from build123d import *

# Parameters (mm, degrees)
F0_R     = 4.7625
F0_R_2   = 1.27
F1_DEPTH = 3.175
F2_R     = 12.7


with BuildPart() as f1:
    # F0 (on Front) → F1 (new body, symmetric)
    with BuildSketch(Plane.XZ):
        with BuildLine():
            ThreePointArc((-58.739439, 25.245564), (-67.461813, 27.891467), (-61.679409, 20.845588))
            ThreePointArc((-61.679409, 20.845588), (-59.542065, 22.599661), (-58.739439, 25.245564))
        make_face()
        Polygon((-45.276641, -18.754199), (0, 0), (0, 80.759988), (-139.00587, 23.181871), (-110.452903, -45.75109), align=None)
        with Locations((-91.447397, -8.667692)):
            Circle(F0_R, mode=Mode.SUBTRACT)
        with Locations((-96.914986, 4.532236)):
            Circle(F0_R_2, mode=Mode.SUBTRACT)
        with BuildLine():
            ThreePointArc((-56.764349, 12.045635), (-56.978383, 11.340061), (-57.548342, 10.872308))
            ThreePointArc((-57.548342, 10.872308), (-59.207676, 11.559627), (-58.520357, 13.218962))
            ThreePointArc((-58.520357, 13.218962), (-57.328775, 13.101602), (-56.764349, 12.045635))
        make_face(mode=Mode.SUBTRACT)
        with BuildLine():
            ThreePointArc((-58.739439, 25.245564), (-59.542065, 22.599661), (-61.679409, 20.845588))
            ThreePointArc((-61.679409, 20.845588), (-67.461813, 27.891467), (-58.739439, 25.245564))
        make_face(mode=Mode.SUBTRACT)
        Polygon((0, 80.759988), (0, 0), (110.452903, -45.75109), (139.00587, 23.181871), align=None)
        with Locations((58.034349, 12.045635)):
            Circle(F0_R_2, mode=Mode.SUBTRACT)
        with Locations((91.447397, -8.667692)):
            Circle(F0_R, mode=Mode.SUBTRACT)
        with Locations((96.914986, 4.532236)):
            Circle(F0_R_2, mode=Mode.SUBTRACT)
        with Locations((63.501939, 25.245564)):
            Circle(F0_R, mode=Mode.SUBTRACT)
    extrude(amount=F1_DEPTH, both=True)

    # F2
    f2_edges = [f1.edges().sort_by_distance(p)[0] for p in [
        (-139.00587, 0, 23.181871),
        (0, 0, 80.759988),
        (0, 0, 0),
        (110.452903, 0, -45.75109),
        (139.00587, 0, 23.181871),
        (-110.452903, 0, -45.75109),
    ]]
    fillet(f2_edges, radius=F2_R)


solid = f1.part
For this review, take the finished solid that the model builds, in its own axes (mm). A direction names the side the tool comes from. Round coordinates to 2 decimals unless told otherwise and drop trailing zeros. Loops run counter-clockwise (first coordinate to the right, second up) from the corner with the lowest first, then second, coordinate; pieces in that order, holes last. Notation, with made-up numbers: (32.25, 9) - (57.25, 9) arc R24 ccw to (57.25, 46) - close; hole circle Ø11 at (43, 52). An arc over 180 degrees is marked (long way). Put each result on its own line as item: value. Start each with the question number.
1. Consider section B-B on z = 37.5. State the section outline as (x, y) points (3 decimals), plus the area to 3 significant figures.
2. Insertion check: P1, Ø1.5, axis at x = -96.91, z = 4.53, coming from the -Y side; P2, Ø12.5, axis at x = -63.5, z = 25.25, coming from the -Y side (3 decimals); P3, Ø1.5, axis at x = 59.5, y = 0.5, coming from the +Z side; P4, Ø1.5, axis at y = -0.5, z = 65.5, coming from the -X side. Each pin has a flat end and moves straight along its axis. Give the tip position at first contact, or say it passes through.
3. For faces 5 (the cylindrical face through (-134.2, 0.04, 21.04)), 6 (the flat face through (51.13, -0.04, -21.18)), list the 3-axis set-ups (+Z, -Z, +X, -X, +Y, -Y) from which the entire face can be reached by the end or side of a thin tool; tool diameter is ignored.
4. For probe 1 along X at (y, z) = (2.5, -5); probe 2 along X at (y, z) = (0.5, -22); probe 3 along Z at (x, y) = (9.5, 2), list the stretches that pass through material, from the lowest coordinate up. Write a range as [from, to].
5. Consider section C-C on x = 48. State the section outline as (y, z) points (3 decimals), plus the area to 3 significant figures.
6. Mouldability with a two-part tool opening along X and no side actions: class faces 1 (the cylindrical face through (-0.07, -0.044, -1.047)), 2 (the flat face through (-65.21, -0.04, 53.75)), 3 (the cylindrical face through (-108.31, 0.044, -40.944)), 4 (the flat face through (-2, -3.175, 20)) as +X half, -X half, draft (parallel to the pull), parting line (faces both ways), or undercut.
7. Consider section A-A on y = 0.75. State how many separate pieces and enclosed holes the cut face has, plus the area to 3 significant figures.
Result sheet:
1. outline: (-104.439, -3.175) - (104.439, -3.175) - (104.439, 3.175) - (-104.439, 3.175) - close
1. area: 1,330 mm^2
2. P1: through
2. P2: y = -3.175
2. P3: z = 56.42
2. P4: x = -38.65
3. face 5: -X, +Y, -Y
3. face 6: -Z, +Y, -Y
4. probe 1: [-127.33, -94.49], [-88.41, -12.07], [12.07, 88.41], [94.49, 127.33]
4. probe 2: [-120.29, -53.11], [53.11, 120.29]
4. probe 3: [-3.94, 76.82]
5. outline: (-3.175, -19.882) - (3.175, -19.882) - (3.175, 60.878) - (-3.175, 60.878) - close
5. area: 513 mm^2
6. face 1: undercut
6. face 2: -X half
6. face 3: undercut
6. face 4: draft
7. separate pieces: 1
7. enclosed holes: 8
7. area: 19,700 mm^2
